Here's how the part is built. I have some questions about the finished solid (model axes, mm). Face numbers are marked on the shaded views. A direction names the side the tool comes from. Give positions to 0.01 mm unless a question says otherwise; leave off trailing zeros.
Q1. For the marked faces 4 and 5, which set-ups out of +Z, -Z, +X, -X, +Y, -Y let a thin tool reach every point of the face, with its end or its side?
Q2. I need wall thicknesses on probe 1 along Z at (x, y) = (-75.5, 32). Which ranges of the line are inside material? Lowest first, please.
Q3. Thinking about a two-plate mould opening in Y: for the marked faces 1, 2 and 3, which applies, pulls with the +Y half, pulls with the -Y half, needs draft (parallel to the pull), parting line crosses it, or undercut?
Q4. I'm going to push a flat-ended pin straight in: P1, Ø5.5, axis at x = -82.28, y = 38.1, coming from the +Z side. Where does the tip first touch, or does it pass through?
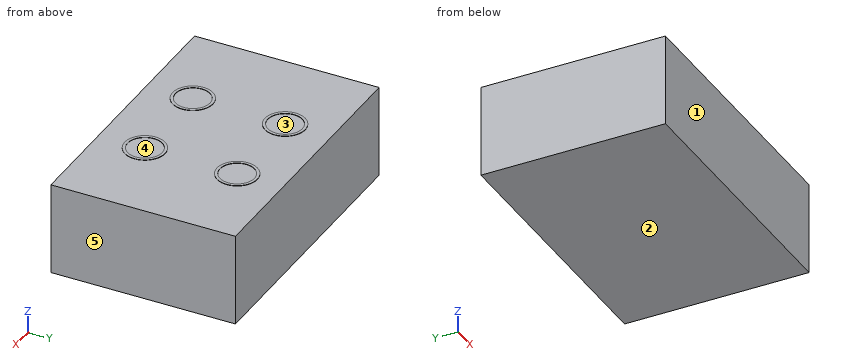
```python
from build123d import *

# Parameters (mm, degrees)
F0_W     = 76.2
F0_H     = 50.8
F1_DEPTH = 25.4
F2_R     = 5.55625
F3_DEPTH = 0.1
F4_R     = 4.7625
F5_DEPTH = 0.1


with BuildPart() as f1:
    # F0 (on Top) → F1 (new body)
    with BuildSketch(Plane.XY):
        with Locations((-94.978769, 25.4)):
            Rectangle(F0_W, F0_H)
    extrude(amount=-F1_DEPTH)

    # F2 (on face) → F3 (join)
    with BuildSketch(Plane.XY):
        with Locations((-107.678769, 38.1)):
            Circle(F2_R)
        with Locations((-82.278769, 38.1)):
            Circle(F2_R)
        with Locations((-107.678769, 12.7)):
            Circle(F2_R)
        with Locations((-82.278769, 12.7)):
            Circle(F2_R)
    extrude(amount=F3_DEPTH)

    # F4 (on face) → F5 (cut)
    with BuildSketch(Plane.XY.offset(0.1)):
        with Locations((-107.678769, 38.091734)):
            Circle(F4_R)
        with Locations((-82.278769, 38.1)):
            Circle(F4_R)
        with Locations((-107.678769, 12.7)):
            Circle(F4_R)
        with Locations((-82.278769, 12.7)):
            Circle(F4_R)
    extrude(amount=-F5_DEPTH, mode=Mode.SUBTRACT)


solid = f1.part
```
Solutions:
1. face 4: +Z
1. face 5: +Z, -Z, +X, +Y, -Y
2. probe 1: z = -25.4 to 0
3. face 1: pulls with the -Y half
3. face 2: needs draft
3. face 3: undercut
4. P1: stops at z = 0
